The model under review builds one solid part; all positions refer to its coordinate system, in mm. A direction names the side the tool comes from. Coordinates: 2 decimals unless noted, no trailing zeros. Loops run counter-clockwise (first coordinate to the right, second up) from the corner with the lowest first, then second, coordinate; pieces in that order, holes last. Notation, with made-up numbers: M 8.25,10 L 31.25,10 A23 cw 31.25,19 Z; hole C 73,1 d4. An arc over 180 degrees is marked long. Use one line per item in the form item = value.
```python
from build123d import *

# Parameters (mm, degrees)
PAD_DEPTH = 9


with BuildPart() as part:
    # Sketch → Pad (new body)
    with BuildSketch(Plane.XY):
        Polygon((-1, 50), (-50, 50), (-50, -2), (-2, -2), (-2, -66), (66, -66), (66, -0.666667), (114.8, 64.4), (47.6, 114.8), align=None)
        Polygon((0, 48), (48, 112), (112, 64), (64, 0), (64, -64), (0, -64), (0, 0), (-48, 0), (-48, 48), align=None, mode=Mode.SUBTRACT)
    extrude(amount=PAD_DEPTH)


solid = part.part
```
1. Insertion check: P1, Ø5, axis at y = -27, z = 4, coming from the -X side; P2, Ø5, axis at y = 50.5, z = 2, coming from the +X side; P3, Ø2.5, axis at x = -21, z = 6, coming from the +Y side; P4, Ø3, axis at x = -5, y = -3, coming from the -Z side. Each pin has a flat end and moves straight along its axis. Give the tip position at first contact, or say it passes through.
Response values:
P1 = -2
P2 = 106.25
P3 = 50
P4 = 0
2. The part is to be moulded in two halves that separate along X. For faces 4 (the face through (0, -32, 4)), 5 (the face through (1, 52, 9)), 6 (the face through (66, -34, 4)), say which applies: pulls with the +X half, pulls with the -X half, needs draft (parallel to the pull), parting line crosses it, or undercut.
Response values:
face_4 = undercut
face_5 = needs draft
face_6 = pulls with the +X half
3. Add section B-B (y = -41). State the section outline as (x, z) points, then the cut area to 3 significant figures.
Response values:
outline = M -2,0 L 0,0 L 0,9 L -2,9 Z; M 64,0 L 66,0 L 66,9 L 64,9 Z
area = 36.0 mm^2
4. Add section A-A (x = -35.5). State the section outline as (y, z) points, then the cut area to 3 significant figures.
Response values:
outline = M -2,0 L 0,0 L 0,9 L -2,9 Z; M 48,0 L 50,0 L 50,9 L 48,9 Z
area = 36.0 mm^2
5. Machinability: for faces 1 (the face through (-24, 0, 4)), 2 (the face through (-25, 50, 4)), 3 (the face through (-2, -34, 4)), which of the approach directions +Z, -Z, +X, -X, +Y, -Y give a long, thin tool a straight path to every point of the face, cutting with its end or side? Answer none if there is none.
Response values:
face_1 = +Z, -Z
face_2 = +Z, -Z, -X, +Y
face_3 = +Z, -Z, -X, -Y
6. Add section C-C (z = 4.75). State the section outline as (x, y) points.
Response values:
outline = M -50,-2 L -2,-2 L -2,-66 L 66,-66 L 66,-0.67 L 114.8,64.4 L 47.6,114.8 L -1,50 L -50,50 Z; hole M -48,0 L 0,0 L 0,-64 L 64,-64 L 64,0 L 112,64 L 48,112 L 0,48 L -48,48 Z
7. Wall thickness on line 1 along Y through (x, z) = (-28.5, 5.75); line 2 along X through (y, z) = (-3.5, 0.75); line 3 along X through (y, z) = (39, 4): over which ranges is each line inside the solid? List them lowest first. Write a range as from..to.
Response values:
line_1 = -2..0, 48..50
line_2 = -2..0, 64..66
line_3 = -50..-48, 93.25..95.75
